Design review of the part built by this model. Coordinates are the model's own, in mm. A direction names the side the tool comes from. Give positions to 0.01 mm unless a question says otherwise; leave off trailing zeros. Loops run counter-clockwise (first coordinate to the right, second up) from the corner with the lowest first, then second, coordinate; pieces in that order, holes last. Notation, with made-up numbers: M 83,68 L 89,68 A18 cw 89,95 Z; hole C -5,16.5 d7. An arc over 180 degrees is marked long. Use CSV: the item, a comma, the result in double quotes.
from build123d import *

# Parameters (mm, degrees)
BOSS_EXTRUDE4_DEPTH      = 70
CUT_EXTRUDE7_DEPTH       = 70
CUT_EXTRUDE8_DEPTH       = 70
CUT_EXTRUDE9_DEPTH       = 70
CUT_EXTRUDE10_DEPTH      = 70
SKETCH9_W                = 19.742548684
SKETCH9_H                = 10.626968924
CUT_EXTRUDE11_DEPTH      = 70
SKETCH10_W               = 30.173725447
SKETCH10_H               = 4.529281074
BOSS_EXTRUDE6_DEPTH      = 20
BOSS_EXTRUDE6_DEPTH_BACK = 20
SKETCH11_W               = 30.173725447
SKETCH11_H               = 4.529281074
BOSS_EXTRUDE7_DEPTH      = 20
BOSS_EXTRUDE7_DEPTH_BACK = 20
SKETCH12_W               = 12.373535054
SKETCH12_H               = 7.384206403
CUT_EXTRUDE12_DEPTH      = 60


with BuildPart() as part:
    # Sketch1 → Boss-Extrude4 (new body)
    with BuildSketch(Plane(origin=(0, 0, 0), x_dir=(0, 0, -1), z_dir=(1, 0, 0))):
        with BuildLine():
            Line((-39.22009442, -23.730076692), (-9.22009442, -23.730076692))
            ThreePointArc((-9.22009442, -23.730076692), (-30.130831643, 17.067070654), (-73.745048282, 31.190323456))
            ThreePointArc((-73.745048282, 31.190323456), (-77.395108799, 29.973959621), (-80.055244789, 27.19436266))
            Line((-80.055244789, 27.19436266), (-80.119694314, 21.843458315))
            Line((-80.119694314, 21.843458315), (-111.566080144, 41.091665162))
            ThreePointArc((-111.566080144, 41.091665162), (-114.864867075, 40.185656866), (-114.171074211, 36.835806464))
            Line((-114.171074211, 36.835806464), (-113.899114734, 36.669341157))
            Line((-113.899114734, 36.669341157), (-77.842344496, 14.599136476))
            ThreePointArc((-77.842344496, 14.599136476), (-46.303479727, 7.755753907), (-39.22009442, -23.730076692))
        make_face()
    extrude(amount=-BOSS_EXTRUDE4_DEPTH)

    # Sketch7 → Cut-Extrude7 (cut)
    with BuildSketch(Plane(origin=(0, -19.784860197, 12.110233703), x_dir=(1, 0, 0), z_dir=(0, 0.8529078546066994, -0.5220614825384052))):
        Polygon((-70, -137.087313056), (0, -134.019745414), (0, -116.607961697), (-70, -116.607961697), align=None)
        with BuildLine():
            Line((0, -116.607961697), (0, -93.251406208))
            ThreePointArc((0, -93.251406208), (-14.740425592, -110.265300978), (-36.339578744, -116.607961697))
            Line((-36.339578744, -116.607961697), (0, -116.607961697))
        make_face()
        with BuildLine():
            Line((-70, -116.607961697), (-36.339578744, -116.607961697))
            ThreePointArc((-36.339578744, -116.607961697), (-55.528547719, -111.697453308), (-70, -98.173153259))
            Line((-70, -98.173153259), (-70, -116.607961697))
        make_face()
    extrude(amount=-CUT_EXTRUDE7_DEPTH, mode=Mode.SUBTRACT)

    # 3DSketch2 → Cut-Extrude8 (cut)
    with BuildSketch(Plane(origin=(-19.171968763, -23.730076692, 9.22009442), x_dir=(-0.9120096253806464, 0.410168798439195, 0), z_dir=(0, 0, 1))):
        Polygon((0, 0), (33.948715461, 15.26815446), (40.815441858, 0), (6.866726397, -15.26815446), align=None)
    extrude(amount=CUT_EXTRUDE8_DEPTH, mode=Mode.SUBTRACT)

    # 3DSketch3 → Cut-Extrude9 (cut)
    with BuildSketch(Plane(origin=(-47.927611425, 14.599136476, 77.842344496), x_dir=(0.6530368290826427, 0, -0.7573261515765103), z_dir=(0, -1, 0))):
        Polygon((0, 0), (25.318083545, -21.831599189), (44.143312647, 0), (18.825229102, 21.831599189), align=None)
    extrude(amount=-CUT_EXTRUDE9_DEPTH, mode=Mode.SUBTRACT)

    # 3DSketch4 → Cut-Extrude10 (cut, along a direction that is not the sketch's normal)
    with BuildSketch(Plane(origin=(-19.22654119, 27.19436266, 80.055244789), x_dir=(-0.9162575030272925, 0.13334663681048042, -0.37774444085588477), z_dir=(0.12328082078814585, 0.9910694599529005, 0.050824844067318485))):
        Polygon((0, 0), (4.481258703, -10.967695522), (31.324240337, 0), (26.842981633, 10.967695522), align=None)
    extrude(amount=-CUT_EXTRUDE10_DEPTH, dir=(0, 1, 0), mode=Mode.SUBTRACT)

    # Sketch9 → Cut-Extrude11 (cut)
    with BuildSketch(Plane(origin=(3.531999691, 28.394173594, 1.456133504), x_dir=(-0.9923718250866462, 0.12311902997688387, 0.006313891965344148), z_dir=(-0.12328082078814556, -0.9910694599529005, -0.05082484406731809))):
        with Locations((33.130862907, -73.819623484)):
            Rectangle(SKETCH9_W, SKETCH9_H)
    extrude(amount=-CUT_EXTRUDE11_DEPTH, mode=Mode.SUBTRACT)

    # Sketch10 → Boss-Extrude6 (add, two sides)
    with BuildSketch(Plane(origin=(0, 0, 0), x_dir=(0, 0, -1), z_dir=(1, 0, 0))) as boss_extrude6_sk:
        with Locations((-24.133231697, -25.994717229)):
            Rectangle(SKETCH10_W, SKETCH10_H)
    extrude(amount=BOSS_EXTRUDE6_DEPTH)
    extrude(boss_extrude6_sk.sketch, amount=-BOSS_EXTRUDE6_DEPTH_BACK)

    # Sketch11 → Boss-Extrude7 (add, two sides)
    with BuildSketch(Plane.ZY.offset(70)) as boss_extrude7_sk:
        with Locations((24.133231697, -25.994717229)):
            Rectangle(SKETCH11_W, SKETCH11_H)
    extrude(amount=BOSS_EXTRUDE7_DEPTH)
    extrude(boss_extrude7_sk.sketch, amount=-BOSS_EXTRUDE7_DEPTH_BACK)

    # Sketch12 → Cut-Extrude12 (cut)
    with BuildSketch(Plane(origin=(0, 0, 9.046368973), x_dir=(-1, 0, 0), z_dir=(0, 0, -1))):
        with Locations((50.666491964, -27.012348263)):
            Rectangle(SKETCH12_W, SKETCH12_H)
    extrude(amount=-CUT_EXTRUDE12_DEPTH, mode=Mode.SUBTRACT)


solid = part.part
(1) We need section C-C on z = 30.5. State the section outline as (x, y) points, then the cut area to 3 significant figures.
A:
outline,"M -90,-28.26 L -56.85,-28.26 L -56.85,-23.32 L -56.4,-23.32 L -56.4,-6.99 L -19.17,-6.99 L -19.17,-23.73 L -20,-23.73 L -20,-28.26 L 20,-28.26 L 20,-23.73 L 0,-23.73 L 0,17.38 L -70,17.38 L -70,-23.73 L -90,-23.73 Z"
area,"2,590 mm²"
(2) We need section B-B on x = -61. State the section outline as (y, z) points.
A:
outline,"M -28.26,9.05 L -23.73,9.05 L -23.73,9.22 A60 ccw 31.19,73.75 A8 ccw 27.19,80.06 L 21.84,80.12 L 36.64,104.3 L 32.39,106.9 L 14.6,77.84 A30 cw -23.73,39.22 L -28.26,39.22 Z"
(3) Machinability: for faces 1 (the flat face through (-33, 14.599, 51)), 2 (the cylindrical face through (-9.64, 30, 77.35)), 3 (the flat face through (-19.1, 23, 61)), which of the approach directions +Z, -Z, +X, -X, +Y, -Y give a long, thin tool a straight path to every point of the face, cutting with its end or side? Answer none if there is none.
A:
face 1,"+Z, +Y"
face 2,"+X, -X, +Y"
face 3,"+Y"
(4) Wall thickness on line 1 along Y through (x, z) = (5.5, 22); line 2 along Z through (x, y) = (-74.5, -24); line 3 along Z through (x, y) = (-22, 19): over which ranges is each line inside the solid? List them lowest first. Write a range as [from, to].
A:
line 1,"[-28.26, -23.73]"
line 2,"[9.05, 39.22]"
line 3,"[32.52, 44.41], [80.06, 85.03]"
(5) The part is to be moulded in two halves that separate along X. For faces 4 (the flat face through (0, -26, 9.046)), 5 (the flat face through (0, 4.2, 42.9)), 6 (the flat face through (-70, 10, 45)), 7 (the flat face through (-47.928, 23, 56)), say which applies: released by +X, released by -X, zero draft, split by the parting line, or undercut.
A:
face 4,"zero draft"
face 5,"released by +X"
face 6,"released by -X"
face 7,"undercut"
(6) We need section D-D on y = -5. State the section outline as (x, z) points, then the cut area to 3 significant figures.
A:
outline,"M -70,13.87 L 0,13.87 L 0,38.68 L -70,38.68 Z"
area,"1,740 mm²"
(7) Clearance check with flat-ended pins moving along their axes: P1, Ø8, axis at x = -17.5, z = 87, coming from the -Y side; P2, Ø4, axis at x = -53, z = 98, coming from the -Y side; P3, Ø9, axis at x = -36.5, y = 21, coming from the +Z side. State where each tip first meets the part, or that it passes through.
A:
P1,"y = 17.76"
P2,"y = 25.71"
P3,"z = 95.65"
(8) We need section A-A on z = 66.5. State the section outline as (x, y) points.
A:
outline,"M -70,16.45 L -47.93,16.45 L -47.93,31.32 L -70,31.32 Z; M -19.1,16.45 L 0,16.45 L 0,31.32 L -19.1,31.32 Z"
